Autodesk Inventor part; units mm, degrees
ref_plane "spring_XY" through (0, 0, 0) normal (0, 0, 1) x (1, 0, 0)
ref_plane "spring_YZ" through (0, 0, 0) normal (1, 0, 0) x (0, 1, 0)
ref_plane "spring_ZX" through (0, 0, 0) normal (0, 1, 0) x (0, 0, 1)
sketch "_____1" plane through (0, 0, 0) normal (0, 1, 0) x (1, 0, 0)
  line L0 (0, 0) -> (0, 7)
  line L1 (0, 7) -> (3, 7)
  line L2 (3, 7) -> (3, 0)
  line L3 (3, 0) -> (0, 0)
  line L4 (0, 0) -> (0, 7)
revolve "Revolution1" add sketch "_____1" angle 360 about axis through (0, 0, 0) along (0, 0, 1)
sketch "_____2" plane through (0, 0, 0) normal (0, 1, 0) x (1, 0, 0)
  line L0 (0, 0) -> (0, 7)
  line L1 (2.8, 7) -> (3, 6.8)
  line L2 (3, 6.8) -> (3, 7)
  line L3 (3, 7) -> (2.8, 7)
revolve "Revolution2" cut sketch "_____2" angle 360 about axis through (0, 0, 0) along (0, 0, 1)
sketch "_____3" plane through (0, 0, 0) normal (0, 1, 0) x (1, 0, 0)
  line L0 (0, 0) -> (0, 7)
  line L1 (2.8, 0) -> (3, 0)
  line L2 (3, 0) -> (3, 0.2)
  line L3 (3, 0.2) -> (2.8, 0)
revolve "Revolution3" cut sketch "_____3" angle 360 about axis through (0, 0, 0) along (0, 0, 1)
sketch "Sketch4" plane through (0, 0, 0) normal (0, 0, 1) x (1, 0, 0)
  point P0 (0, 0)
hole "Hole1" at (0, 0, 0) direction (0, 0, -1) diameter 3 depth 7
sketch "_____5" plane through (0, 0, 0) normal (0, 1, 0) x (1, 0, 0)
  line L0 (0, -14) -> (0, 14)
  line L1 (1.5, 6.8) -> (1.7, 7)
  line L2 (1.7, 7) -> (1.5, 7)
  line L3 (1.5, 7) -> (1.5, 6.8)
revolve "Revolution4" cut sketch "_____5" angle 360 about axis through (0, 0, 14) along (0, 0, 1)
sketch "_____6" plane through (0, 0, 0) normal (0, 1, 0) x (1, 0, 0)
  line L0 (0, -14) -> (0, 14)
  line L1 (1.5, 0.2) -> (1.5, 0)
  line L2 (1.5, 0) -> (1.7, 0)
  line L3 (1.7, 0) -> (1.5, 0.2)
revolve "Revolution5" cut sketch "_____6" angle 360 about axis through (0, 0, 14) along (0, 0, 1)
ref_plane "spring_XY" through (0, 0, 0) normal (0, 0, 1) x (1, 0, 0)
ref_plane "spring_YZ" through (0, 0, 0) normal (1, 0, 0) x (0, 1, 0)
ref_plane "spring_ZX" through (0, 0, 0) normal (0, 1, 0) x (0, 0, 1)
ref_plane "to_bolt_XY" through (0, 0, -7) normal (0, 0, 1) x (1, 0, 0)
ref_plane "to_bolt_YZ" through (0, 0, -7) normal (1, 0, 0) x (0, 1, 0)
ref_plane "to_bolt_ZX" through (0, 0, -7) normal (0, 1, 0) x (0, 0, 1)
properties part number "FWSSA-D6-V3-T7"
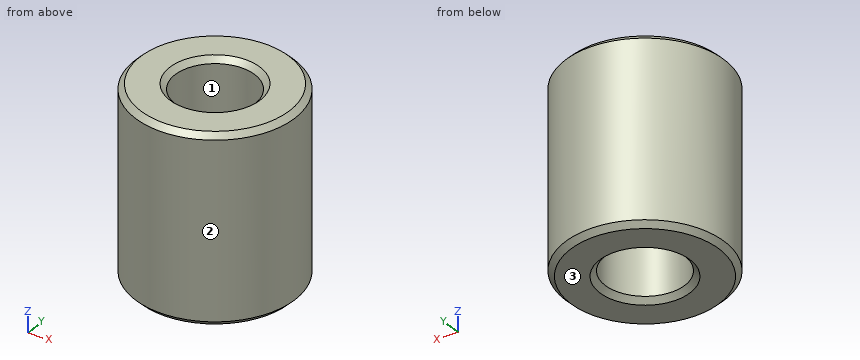
Here's how the part is built. I have some questions about the finished solid (model axes, mm). Face numbers are marked on the shaded views. Round coordinates to 2 decimals unless told otherwise and drop trailing zeros. Order: outer loops, then holes, each group sorted by start corner. A loop starts at its lowest first (then second) coordinate and runs counter-clockwise, first axis right, second up. Notation, with made-up numbers: (81.25, 8) -> (89.25, 8) arc R30 cw to (89.25, 37) -> close; hole circle Ø11 at (-30.75, -33.75). An arc over 180 degrees is marked (long way). Use CSV: the item, a comma, the result in double quotes.
1. I need wall thicknesses on line 1 along Y through (x, z) = (0, -2); line 2 along X through (y, z) = (0.5, -3); line 3 along Y through (x, z) = (-0.7, -3.5). Which ranges of each line are inside material? Lowest first, please.
Recorded:
line 1,"y = -3 to -1.5, 1.5 to 3"
line 2,"x = -2.96 to -1.41, 1.41 to 2.96"
line 3,"y = -2.92 to -1.33, 1.33 to 2.92"
2. I want a section at A-A on y = 0. List the corners of the cut face in (x, z) for me, and give its area (3 significant figures).
Recorded:
outline,"(-3, -6.8) -> (-2.8, -7) -> (-1.7, -7) -> (-1.5, -6.8) -> (-1.5, -0.2) -> (-1.7, 0) -> (-2.8, 0) -> (-3, -0.2) -> close; (1.5, -6.8) -> (1.7, -7) -> (2.8, -7) -> (3, -6.8) -> (3, -0.2) -> (2.8, 0) -> (1.7, 0) -> (1.5, -0.2) -> close"
area,"20.8 mm2"
3. Thinking about a two-plate mould opening in X: for the marked faces 1, 2 and 3, which applies, pulls with the +X half, pulls with the -X half, needs draft (parallel to the pull), parting line crosses it, or undercut?
Recorded:
face 1,"undercut"
face 2,"parting line crosses it"
face 3,"needs draft"
4. I want a section at C-C on z = -1.5. List the corners of the cut face in (x, y) for me, and give its area (3 significant figures).
Recorded:
outline,"circle Ø6 at (0, 0); hole circle Ø3 at (0, 0)"
area,"21.2 mm2"
